```python
from build123d import *

# Parameters (mm, degrees)
EXTRUDE_1_DEPTH     = 59
SKETCH_2_R          = 50
CUT_EXTRUDE_1_DEPTH = 322.653980979


with BuildPart() as part:
    # 草图1 → 凸台-拉伸1 (new body)
    with BuildSketch(Plane.XY):
        with BuildLine():
            Line((-60, 150.111069989), (-60, 175))
            ThreePointArc((-60, 175), (0, 235), (60, 175))
            Line((60, 175), (60, 150.111069989))
            ThreePointArc((60, 150.111069989), (86.794919243, 50.111069989), (160, -23.094010768))
            Line((160, -23.094010768), (181.554445662, -35.538475773))
            ThreePointArc((181.554445662, -35.538475773), (203.515969889, -117.5), (121.554445662, -139.461524227))
            Line((121.554445662, -139.461524227), (100, -127.017059222))
            ThreePointArc((100, -127.017059222), (0, -100.222139979), (-100, -127.017059222))
            Line((-100, -127.017059222), (-121.554445662, -139.461524227))
            ThreePointArc((-121.554445662, -139.461524227), (-203.515969889, -117.5), (-181.554445662, -35.538475773))
            Line((-181.554445662, -35.538475773), (-160, -23.094010768))
            ThreePointArc((-160, -23.094010768), (-86.794919243, 50.111069989), (-60, 150.111069989))
        make_face()
    extrude(amount=EXTRUDE_1_DEPTH)

    # 草图2 → 切除-拉伸1 (cut, through all)
    with BuildSketch(Plane.XY.offset(59)):
        with Locations((-151.554445662, -87.5)):
            Circle(SKETCH_2_R)
        with Locations((0, 175)):
            Circle(SKETCH_2_R)
        with Locations((151.554445662, -87.5)):
            Circle(SKETCH_2_R)
    extrude(amount=-CUT_EXTRUDE_1_DEPTH, mode=Mode.SUBTRACT)


solid = part.part
```
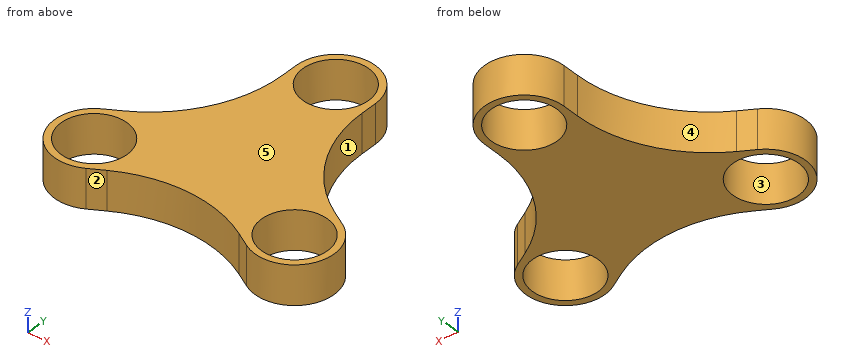
Build history of the part. All positions in model axes, mm. Face numbers are marked on the shaded views. A direction names the side the tool comes from. Give positions to 0.01 mm unless a question says otherwise; leave off trailing zeros. Order: outer loops, then holes, each group sorted by start corner. A loop starts at its lowest first (then second) coordinate and runs counter-clockwise, first axis right, second up. Notation, with made-up numbers: M -26.5,19 L 20.5,19 A22 cw 20.5,38 Z; hole C 31,50.25 d6. An arc over 180 degrees is marked long. Write item = value, one per line. Start each with the question number.
(1) Slice it at C-C on y = 195.5. Write the cut outline in (x, z).
(2) Slice it at D-D on y = -9.5. Write the cut outline in (x, z), plus the area to 3 significant figures.
(3) Which spindle directions (+Z, -Z, +X, -X, +Y, -Y) get a long thin tool onto all of the face, cutting with end or side? Do the marked faces 1 and 2. Say none if no direction does.
(4) Pin check, flat tips, straight feed: pin 1 Ø7.5 at (y, z) = (161.5, 23) entering from -X; pin 2 Ø10 at (x, z) = (-17, 42) entering from +Y; pin 3 Ø8 at (y, z) = (11, 10) entering from +X. Stop position of each tip, or through.
(5) Slice it at A-A on x = 0. Write the cut outline in (y, z).
(6) Two-plate mould, pull along X, no slides. Class the marked faces 3, 4 and 5: released by +X, released by -X, zero draft, split by the parting line, or undercut.
(7) Slice it at B-B on y = -87.5. Write the cut outline in (x, z).
(8) Probe L1, parallel to X at y = -87, z = 23; L2, parallel to Y at x = 0, z = 29; L3, parallel to X at y = -126, z = 20. List the from-to ranges inside material, lowest first. Write a range as [from, to].
Responses:
q1.outline = M -56.39,0 L -45.6,0 L -45.6,59 L -56.39,59 Z; M 45.6,0 L 56.39,0 L 56.39,59 L 45.6,59 Z
q2.outline = M -139.48,0 L 139.48,0 L 139.48,59 L -139.48,59 Z
q2.area = 16,500 mm2
q3.face_1 = +Z, -Z, +X, +Y
q3.face_2 = +Z, -Z, -Y
q4.pin_1 = -60
q4.pin_2 = 233.79
q4.pin_3 = 120.29
q5.outline = M -100.22,0 L 125,0 L 125,59 L -100.22,59 Z; M 225,0 L 235,0 L 235,59 L 225,59 Z
q6.face_3 = undercut
q6.face_4 = released by -X
q6.face_5 = zero draft
q7.outline = M -211.55,0 L -201.55,0 L -201.55,59 L -211.55,59 Z; M -101.55,0 L 101.55,0 L 101.55,59 L -101.55,59 Z; M 201.55,0 L 211.55,0 L 211.55,59 L 201.55,59 Z
q8.L1 = [-211.55, -201.55], [-101.56, 101.56], [201.55, 211.55]
q8.L2 = [-100.22, 125], [225, 235]
q8.L3 = [-197.57, -183.46], [-119.65, -98.22], [98.22, 119.65], [183.46, 197.57]
